The listing builds one solid part. Answer for the finished solid, in the listing's coordinates (mm). Face numbers are marked on the shaded views. A direction names the side the tool comes from. Coordinates: 2 decimals unless noted, no trailing zeros. Loops run counter-clockwise (first coordinate to the right, second up) from the corner with the lowest first, then second, coordinate; pieces in that order, holes last. Notation, with made-up numbers: M 40,12 L 57,12 A16 cw 57,17 Z; hole C 69.5,-26.75 d3. An arc over 180 degrees is marked long. Answer in a Markdown table with one row per item. Add a question column.
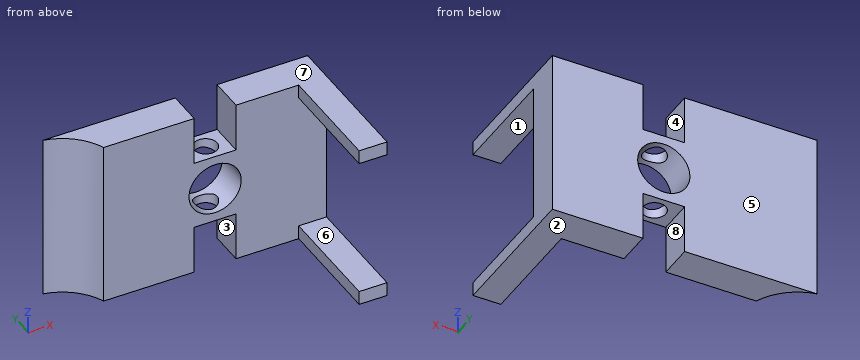
from build123d import *

# Parameters (mm, degrees)
BOSS_EXTRUDE1_DEPTH = 12
CUT_EXTRUDE1_REACH  = 32.712
SKETCH4_R           = 1.65
SKETCH4_3_W         = 6
SKETCH4_3_H         = 5
SKETCH4_3_R         = 1.65
CUT_EXTRUDE3_DEPTH  = 7
CUT_EXTRUDE2_REACH  = 25.022
SKETCH5_R           = 3.75
SKETCH6_W           = 4
SKETCH6_H           = 16
BOSS_EXTRUDE2_DEPTH = 24
CUT_EXTRUDE4_REACH  = 42.525
SKETCH7_W           = 20
SKETCH7_H           = 16


with BuildPart() as part:
    # Sketch3 → Boss-Extrude1 (new, symmetric)
    with BuildSketch(Plane.XY):
        with BuildLine():
            Line((-13, -2.5), (19, -2.5))
            Line((19, -2.5), (19, 2.5))
            Line((19, 2.5), (-19, 2.5))
            ThreePointArc((-19, 2.5), (-15.348369117, 0.781957059), (-13, -2.5))
        make_face()
    extrude(amount=BOSS_EXTRUDE1_DEPTH, both=True)

    # Sketch4 → Cut-Extrude1 (cut, up to next)
    with BuildSketch(Plane.XY.offset(12), mode=Mode.PRIVATE) as cut_extrude1_sk1:
        with Locations((3, 0)):
            Circle(SKETCH4_R)
    cut_extrude1_tool1 = extrude(cut_extrude1_sk1.sketch, amount=-CUT_EXTRUDE1_REACH, mode=Mode.PRIVATE) & part.part
    add(cut_extrude1_tool1.solids().sort_by_distance((3, 0, 12))[0], mode=Mode.SUBTRACT)

    # Sketch4<3> → Cut-Extrude3 (cut)
    with BuildSketch(Plane.XY.offset(12)):
        with Locations((3, 0)):
            Rectangle(SKETCH4_3_W, SKETCH4_3_H)
        with Locations((3, 0)):
            Circle(SKETCH4_3_R, mode=Mode.SUBTRACT)
    cut_extrude3 = extrude(amount=-CUT_EXTRUDE3_DEPTH, mode=Mode.SUBTRACT)

    # Mirror1: Cut-Extrude3 across plane
    add(cut_extrude3.mirror(Plane.XY), mode=Mode.SUBTRACT)

    # Sketch5 → Cut-Extrude2 (cut, up to next)
    with BuildSketch(Plane(origin=(0, 2.5, 0), x_dir=(1, 0, 0), z_dir=(0, 1, 0)), mode=Mode.PRIVATE) as cut_extrude2_sk1:
        with Locations(Location((3, 0, 0), (0, 0, 270))):
            Circle(SKETCH5_R)
    cut_extrude2_tool1 = extrude(cut_extrude2_sk1.sketch, amount=-CUT_EXTRUDE2_REACH, mode=Mode.PRIVATE) & part.part
    add(cut_extrude2_tool1.solids().sort_by_distance((3, 2.5, 0))[0], mode=Mode.SUBTRACT)

    # Sketch6 → Boss-Extrude2 (add)
    with BuildSketch(Plane.XY.offset(12)):
        with Locations((17, -10.5)):
            Rectangle(SKETCH6_W, SKETCH6_H)
    extrude(amount=-BOSS_EXTRUDE2_DEPTH)

    # Sketch7 → Cut-Extrude4 (cut, up to next)
    with BuildSketch(Plane.ZY.offset(-15), mode=Mode.PRIVATE) as cut_extrude4_sk1:
        with Locations((0, -10.5)):
            Rectangle(SKETCH7_W, SKETCH7_H)
    cut_extrude4_tool1 = extrude(cut_extrude4_sk1.sketch, amount=-CUT_EXTRUDE4_REACH, mode=Mode.PRIVATE) & part.part
    add(cut_extrude4_tool1.solids().sort_by_distance((15, -10.5, 0))[0], mode=Mode.SUBTRACT)


solid = part.part
(1) A cutting plane is placed at B-B (x = 3). Give the vertices of the cut face in (y, z), plus the area to 3 significant figures.
(2) A cutting plane is placed at C-C (y = -8.5). Give the vertices of the cut face in (x, z).
(3) The mould has two halves that part along Z. Classify the marked faces 1, 2 and 3: released by +Z, released by -Z, zero draft, split by the parting line, or undercut.
(4) Straight lines are drawn through the part: line 1 (Y direction, x = 3, z = -4.2); line 2 (Y direction, x = 7.5, z = 9.5); line 3 (X direction, y = 0, z = 3.75). For each, find the intervals that lie inside material, in ascending order.
(5) A cutting plane is placed at A-A (z = 0). Give the vertices of the cut face in (x, y).
(6) Each of these flat-tipped pins is pushed along its axis until it touches: pin 1 (2 mm diameter, centred on y = -10, z = -11.5, fed in from -X); pin 2 (4.5 mm diameter, centred on x = 3, y = 0, fed in from -Z); pin 3 (8.5 mm diameter, centred on x = 3, z = 0, fed in from -Y); pin 4 (2 mm diameter, centred on x = 3, y = 0, fed in from +Z). Where does it stop, or does it pass through?
(7) A cutting plane is placed at D-D (y = 0). Give the vertices of the cut face in (x, z).
(8) For the marked faces 4, 5, 6, 7 and 8, determine the directions among +Z, -Z, +X, -X, +Y, -Y from which every point of the face is accessible in a straight line to the end or side of a thin tool.
Solved:
| question | item | result |
|---|---|---|
| 1 | outline | M -2.5,-5 L -1.65,-5 L -1.65,-3.75 L -2.5,-3.75 Z; M -2.5,3.75 L -1.65,3.75 L -1.65,5 L -2.5,5 Z; M 1.65,-5 L 2.5,-5 L 2.5,-3.75 L 1.65,-3.75 Z; M 1.65,3.75 L 2.5,3.75 L 2.5,5 L 1.65,5 Z |
| 1 | area | 4.25 mm² |
| 2 | outline | M 15,-12 L 19,-12 L 19,-10 L 15,-10 Z; M 15,10 L 19,10 L 19,12 L 15,12 Z |
| 3 | face 1 | undercut |
| 3 | face 2 | released by -Z |
| 3 | face 3 | zero draft |
| 4 | line 1 | y = -2.5 to -1.65, 1.65 to 2.5 |
| 4 | line 2 | y = -2.5 to 2.5 |
| 4 | line 3 | x = -14.53 to 1.35, 4.65 to 19 |
| 5 | outline | M -19,2.5 A8 cw -13,-2.5 L -0.75,-2.5 L -0.75,2.5 Z; M 6.75,-2.5 L 19,-2.5 L 19,2.5 L 6.75,2.5 Z |
| 6 | pin 1 | stops at x = 15 |
| 6 | pin 2 | stops at z = -5 |
| 6 | pin 3 | stops at y = -2.5 |
| 6 | pin 4 | passes through |
| 7 | outline | M -14.53,-12 L 0,-12 L 0,-5 L 1.35,-5 L 1.35,-3.37 A3.75 cw 1.35,3.37 L 1.35,5 L 0,5 L 0,12 L -14.53,12 Z; M 4.65,-5 L 6,-5 L 6,-12 L 19,-12 L 19,12 L 6,12 L 6,5 L 4.65,5 L 4.65,3.37 A3.75 cw 4.65,-3.37 Z |
| 8 | face 4 | +Z, +Y, -Y |
| 8 | face 5 | +Z, -Z, +X, -X, +Y |
| 8 | face 6 | +X, -X, -Y |
| 8 | face 7 | +Z, +X, -X, +Y, -Y |
| 8 | face 8 | -Z, +Y, -Y |
